Can you work these out from the model? Positions are in its coordinate system, mm. Face numbers are marked on the shaded views. A direction names the side the tool comes from. Round coordinates to 2 decimals unless told otherwise and drop trailing zeros. Loops run counter-clockwise (first coordinate to the right, second up) from the corner with the lowest first, then second, coordinate; pieces in that order, holes last. Notation, with made-up numbers: (1, -0.75) -> (36, -0.75) arc R31 cw to (36, 23.25) -> close; hole circle Ø11 at (-11, 12.5). An arc over 180 degrees is marked (long way). Answer as a JSON object with one key per item and string values.
Solid Edge part; units mm, degrees
sketch "Sketch1" plane through (0, 0, 0) normal (0, -1, 0) x (1, 0, 0)
  arc A0 (5.4852, 7.625) -> (5.4852, -7.625) centre (34.5, 0) ccw
  line L0 (6, -7.625) -> (5.4852, -7.625)
  line L1 (6, -8.625) -> (6, -7.625)
  line L2 (0, -8.625) -> (6, -8.625)
  line L3 (0, 8.625) -> (0, -8.625)
  line L4 (0, 8.625) -> (6, 8.625)
  line L5 (6, 8.625) -> (6, 7.625)
  line L6 (6, 7.625) -> (5.4852, 7.625)
revolve "RevolvedProtrusion1" add sketch "Sketch1" angle 360 about axis through (0, 0, 8.625) along (0, 0, -1)
hole "Hole1" at (0, 0, 8.625) direction (0, 0, -1) diameter 4 end up to next
sketch "Sketch2" plane through (0, 0, 8.625) normal (0, 0, 1) x (1, 0, 0)
  circle A0 centre (0, 0) radius 4
extrude "VaciadoExtruido_1" cut sketch "Sketch2" against normal blind 4
mirror "Mirror1" about plane through (0, 0, 0) normal (0, 0, 1) of "VaciadoExtruido_1"
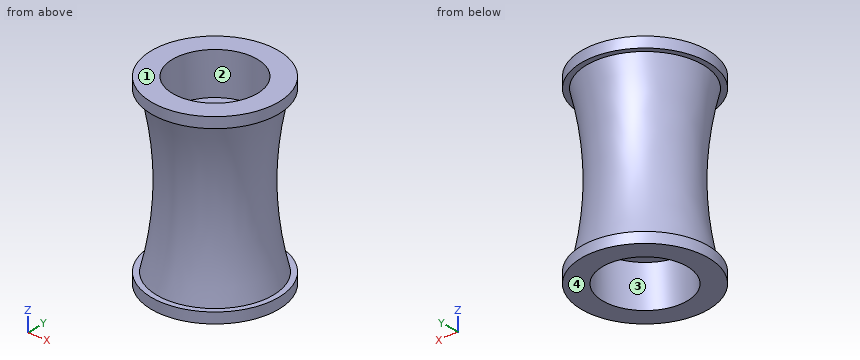
Q1. I want a section at C-C, the plane z = -0.5. Write out the boundary of the cut face in (x, y).
Determined:
{"outline": "circle Ø9.01 at (0, 0); hole circle Ø4 at (0, 0)"}
Q2. I want a section at A-A, the plane x = 0. Write out the boundary of the cut face in (y, z) (3 decimals), then the cut area to 3 significant figures.
Determined:
{"outline": "(-6, -8.625) -> (-4, -8.625) -> (-4, -4.625) -> (-2, -4.625) -> (-2, 4.625) -> (-4, 4.625) -> (-4, 8.625) -> (-6, 8.625) -> (-6, 7.625) -> (-5.485, 7.625) arc R30 cw to (-5.485, -7.625) -> (-6, -7.625) -> close; (2, -4.625) -> (4, -4.625) -> (4, -8.625) -> (6, -8.625) -> (6, -7.625) -> (5.485, -7.625) arc R30 cw to (5.485, 7.625) -> (6, 7.625) -> (6, 8.625) -> (4, 8.625) -> (4, 4.625) -> (2, 4.625) -> close", "area": "70.2 mm²"}
Q3. If I drill on L1, parallel to Z at x = -1, y = -3.75 (3 decimals); L2, parallel to X at y = 0, z = 0; L3, parallel to X at y = 0, z = -3.75, over which ranges is the centre line in solid material (lowest first)? Write a range as [from, to].
Determined:
{"L1": "[-4.625, 4.625]", "L2": "[-4.5, -2], [2, 4.5]", "L3": "[-4.74, -2], [2, 4.74]"}
Q4. On a 3-axis mill with a long thin cutter (end or side, diameter ignored), from which of +Z, -Z, +X, -X, +Y, -Y can I reach the whole of each face in a straight line? I mean the marked faces 3 and 4. Say none if no direction works.
Determined:
{"face 3": "-Z", "face 4": "-Z, +X, -X, +Y, -Y"}
Q5. I want a section at D-D, the plane z = -5.75. Write out the boundary of the cut face in (x, y), then the cut area to 3 significant figures.
Determined:
{"outline": "circle Ø10.11 at (0, 0); hole circle Ø8 at (0, 0)", "area": "30.0 mm²"}
Q6. We'd pull the mould along X, two halves only. Please class the marked faces 1 and 2: pulls with the +X half, pulls with the -X half, needs draft (parallel to the pull), parting line crosses it, or undercut.
Determined:
{"face 1": "needs draft", "face 2": "undercut"}
Q7. I'm going to push flat-ended pins straight in: pin 1 (1 mm diameter, centred on x = -1.5, y = -2.5, fed in from +Z) (3 decimals); pin 2 (5 mm diameter, centred on y = -4, z = 2, fed in from -X); pin 3 (3 mm diameter, centred on x = 4.5, z = -1.5, fed in from -Y); pin 4 (6.5 mm diameter, centred on x = -2, y = 0, fed in from +Z) (3 decimals). Where does each tip first touch, or does it pass through?
Determined:
{"pin 1": "z = 4.625", "pin 2": "x = -4.34", "pin 3": "y = -3.41", "pin 4": "z = 8.625"}
